from build123d import *

# Parameters (mm, degrees)
ESQUISSE1_W        = 26.847127718
ESQUISSE1_H        = 19.360909412
BOSS_EXTRU_1_DEPTH = 5


with BuildPart() as part:
    # Esquisse1 → Boss.-Extru.1 (new body)
    with BuildSketch(Plane(origin=(0, 0, 0), x_dir=(1, 0, 0), z_dir=(0, 1, 0))):
        with Locations((-13.423563859, 9.680454706)):
            Rectangle(ESQUISSE1_W, ESQUISSE1_H)
    extrude(amount=BOSS_EXTRU_1_DEPTH)

    # Esquisse2 → Enlèvement de matière-Révolution1 (revolve, cut)
    with BuildSketch(Plane(origin=(0, 5, 0), x_dir=(1, 0, 0), z_dir=(0, 1, 0))):
        with BuildLine():
            Line((-13.423563859, 12.17807818), (-13.423563859, 7.182831232))
            ThreePointArc((-13.423563859, 7.182831232), (-10.925940385, 9.680454706), (-13.423563859, 12.17807818))
        make_face()
    revolve(axis=Axis((-13.423563859, 5, -17.260196432), (0, 0, 1)), mode=Mode.SUBTRACT)


solid = part.part
For this review, take the finished solid that the model builds, in its own axes (mm). Round coordinates to 2 decimals unless told otherwise and drop trailing zeros. Loops run counter-clockwise (first coordinate to the right, second up) from the corner with the lowest first, then second, coordinate; pieces in that order, holes last. Notation, with made-up numbers: (55, 8) - (114, 8) arc R31 cw to (114, 45) - close; hole circle Ø11 at (70, 21.25). An arc over 180 degrees is marked (long way). One line per question, with ' | ' between items.
Q1. Take a section at B-B (x = -13.75). Give the boundary of the cut face in (y, z), and give its area (3 significant figures).
Taken from the geometry:
outline: (0, -19.36) - (5, -19.36) - (5, -12.16) arc R2.48 cw to (5, -7.2) - (5, 0) - (0, 0) - close | area: 87.2 mm²
Q2. Take a section at C-C (z = -8.75). Give the boundary of the cut face in (x, y).
Taken from the geometry:
outline: (-26.85, 0) - (0, 0) - (0, 5) - (-11.11, 5) arc R2.32 cw to (-15.74, 5) - (-26.85, 5) - close
Q3. For line 1 along Z through (x, y) = (-15, 3.95); line 2 along Z through (x, y) = (-14.75, 3.2); line 3 along Y through (x, z) = (-12, -10.75), list the stretches that pass through material, from the lowest coordinate up. Write a range as [from, to].
Taken from the geometry:
line 1: z = [-19.36, -11.31], [-8.05, 0] | line 2: z = [-19.36, -10.79], [-8.57, 0] | line 3: y = [0, 3.25]
Q4. Take a section at A-A (y = 4.55). Give the boundary of the cut face in (x, z).
Taken from the geometry:
outline: (-26.85, -19.36) - (0, -19.36) - (0, 0) - (-26.85, 0) - close; hole circle Ø4.91 at (-13.42, -9.68)
